from build123d import *

# Parameters (mm, degrees)
SKETCH1_W               = 55.5
SKETCH1_H               = 56
BOSS_EXTRUDE1_DEPTH     = 3
BOSS_EXTRUDE2_DEPTH     = 28
BOSS_EXTRUDE3_DEPTH     = 35
CUT_EXTRUDE3_DEPTH      = 61.495475037
CUT_EXTRUDE3_DEPTH_BACK = 61.495475037
SKETCH6_W               = 15.5
SKETCH6_H               = 56
BOSS_EXTRUDE4_DEPTH     = 0.6
SKETCH7_R               = 7.1
BOSS_EXTRUDE5_DEPTH     = 1.7
FILLET2_R               = 1


with BuildPart() as part:
    # Sketch1 → Boss-Extrude1 (new body)
    with BuildSketch(Plane(origin=(0, 0, 0), x_dir=(1, 0, 0), z_dir=(0, 1, 0))):
        Rectangle(SKETCH1_W, SKETCH1_H)
    extrude(amount=BOSS_EXTRUDE1_DEPTH)

    # Sketch3 → Boss-Extrude2 (add, symmetric)
    with BuildSketch(Plane.XY):
        Polygon((-27.75, 3), (-27.75, 40.8), (27.75, 40.8), (27.75, 3), (24.75, 3), (24.75, 37.8), (-24.75, 37.8), (-24.75, 3), align=None)
    extrude(amount=BOSS_EXTRUDE2_DEPTH, both=True)

    # Sketch4 → Boss-Extrude3 (add, symmetric)
    with BuildSketch(Plane.XY):
        Polygon((27.75, 40.8), (-27.75, 40.8), (-27.75, 37.5), (-27.75, 3), (-24.75, 3), (-24.75, 37.8), (24.75, 37.8), (24.75, 3), (27.75, 3), (27.75, 37.5), align=None)
    extrude(amount=BOSS_EXTRUDE3_DEPTH, both=True)

    # Sketch5 → Cut-Extrude3 (cut, two sides: drawn at the far end of the back side and taken through both)
    with BuildSketch(Plane(origin=(0, 0, 0), x_dir=(0, 0, -1), z_dir=(1, 0, 0)).offset(-CUT_EXTRUDE3_DEPTH_BACK)):
        with BuildLine():
            Line((-10.364011889, 35.8), (10.364011889, 35.8))
            ThreePointArc((10.364011889, 35.8), (6.080263232, 20.66392266), (7.526937591, 5))
            Line((7.526937591, 5), (-7.526937591, 5))
            ThreePointArc((-7.526937591, 5), (-6.080263232, 20.66392266), (-10.364011889, 35.8))
        make_face()
        with BuildLine():
            Line((-35, 37.5), (-35, 3))
            Line((-35, 3), (-28, 3))
            ThreePointArc((-28, 3), (-24.398228699, 21.690939105), (-35, 37.5))
        make_face()
        with BuildLine():
            Line((28, 3), (35, 3))
            Line((35, 3), (35, 37.5))
            ThreePointArc((35, 37.5), (24.398228699, 21.690939105), (28, 3))
        make_face()
    extrude(amount=CUT_EXTRUDE3_DEPTH + CUT_EXTRUDE3_DEPTH_BACK, mode=Mode.SUBTRACT)

    # Sketch6 → Boss-Extrude4 (add)
    with BuildSketch(Plane.XZ):
        Rectangle(SKETCH6_W, SKETCH6_H)
    extrude(amount=BOSS_EXTRUDE4_DEPTH)

    # Sketch7 → Boss-Extrude5 (add)
    with BuildSketch(Plane.XZ.offset(0.6)):
        with Locations(Location((0, 0, 0), (0, 0, 270))):
            Circle(SKETCH7_R)
    extrude(amount=BOSS_EXTRUDE5_DEPTH)

    # Fillet2
    fillet2_edges = [part.edges().sort_by_distance(p)[0] for p in [
        (27.75, 40.8, 0),
        (-27.75, 40.8, 0),
    ]]
    fillet(fillet2_edges, radius=FILLET2_R)


solid = part.part
Design review of the part built by this model. Coordinates are the model's own, in mm. A direction names the side the tool comes from. Coordinates: 2 decimals unless noted, no trailing zeros. Order: outer loops, then holes, each group sorted by start corner. A loop starts at its lowest first (then second) coordinate and runs counter-clockwise, first axis right, second up. Notation, with made-up numbers: (-32, 34.5) -> (-7, 34.5) arc R16 cw to (-7, 55.5) -> close; hole circle Ø11 at (74, 51.5). An arc over 180 degrees is marked (long way). Use one line per item in the form item = value. Start each with the question number.
(1) For faces 1 (the cylindrical face through (5.987, -1.438, -3.817)), 2 (the flat face through (0, 1, -28)), 3 (the flat face through (26, 35.8, 0)), 4 (the cylindrical face through (-26.271, 21.959, -24.454)), 5 (the flat face through (24.75, 21, 8)), list the 3-axis set-ups (+Z, -Z, +X, -X, +Y, -Y) from which the entire face can be reached by the end or side of a thin tool; tool diameter is ignored.
(2) Add section C-C on y = 19. State the section outline as (x, z) points, plus the area to 3 significant figures.
(3) Add section A-A on x = -14.5. State the section outline as (y, z) points.
(4) For probe 1 along Y at (x, z) = (10, -27); probe 2 along Y at (x, z) = (0, -16.5); probe 3 along X at (y, z) = (24, 21), list the stretches that pass through material, from the lowest coordinate up.
(5) Add section B-B on z = 0. State the section outline as (x, y) points.
(6) Insertion check: pin 1 (6 mm diameter, centred on y = 16.5, z = 3.5, fed in from +X); pin 2 (0.7 mm diameter, centred on y = -0.5, z = -3.5, fed in from -X); pin 3 (1.1 mm diameter, centred on x = 10, y = 1, fed in from -Z); pin 4 (1.5 mm diameter, centred on x = -25.5, z = -3.5, fed in from -Y). Each pin has a flat end and moves straight along its axis. Give the tip position at first contact, or say it passes through.
(7) The part is to be moulded in two halves that separate along Y. For faces 6 (the flat face through (0, 40.8, 0)), 7 (the flat face through (-26, 35.8, 0)), 8 (the cylindrical face through (26.229, 21.423, 24.345)), 9 (the flat face through (-18, 0, 0)), say which applies: +Y half, -Y half, draft (parallel to the pull), parting line (faces both ways), or undercut.
(8) Add section D-D on z = -15. State the section outline as (x, y) points.
Answer block:
q1.face_1 = -Y
q1.face_2 = -Z, +X, -X, -Y
q1.face_3 = +X, -X
q1.face_4 = -Z, +X, -X
q1.face_5 = +Z, -Z
q2.outline = (-27.75, -24) -> (-24.75, -24) -> (-24.75, -5.96) -> (-27.75, -5.96) -> close; (-27.75, 5.96) -> (-24.75, 5.96) -> (-24.75, 24) -> (-27.75, 24) -> close; (24.75, -24) -> (27.75, -24) -> (27.75, -5.96) -> (24.75, -5.96) -> close; (24.75, 5.96) -> (27.75, 5.96) -> (27.75, 24) -> (24.75, 24) -> close
q2.area = 217 mm²
q3.outline = (0, -28) -> (3, -28) -> (3, 28) -> (0, 28) -> close; (37.8, -35) -> (40.8, -35) -> (40.8, 35) -> (37.8, 35) -> close
q4.probe_1 = 0 to 3, 37.8 to 40.8
q4.probe_2 = -0.6 to 3, 37.8 to 40.8
q4.probe_3 = -27.75 to -24.75, 24.75 to 27.75
q5.outline = (-27.75, 0) -> (-7.75, 0) -> (-7.75, -0.6) -> (-7.1, -0.6) -> (-7.1, -2.3) -> (7.1, -2.3) -> (7.1, -0.6) -> (7.75, -0.6) -> (7.75, 0) -> (27.75, 0) -> (27.75, 5) -> (24.75, 5) -> (24.75, 3) -> (-24.75, 3) -> (-24.75, 5) -> (-27.75, 5) -> close; (-27.75, 35.8) -> (-24.75, 35.8) -> (-24.75, 37.8) -> (24.75, 37.8) -> (24.75, 35.8) -> (27.75, 35.8) -> (27.75, 39.8) arc R1 ccw to (26.75, 40.8) -> (-26.75, 40.8) arc R1 ccw to (-27.75, 39.8) -> close
q6.pin_1 = 27.75
q6.pin_2 = -7.75
q6.pin_3 = -28
q6.pin_4 = 0
q7.face_6 = +Y half
q7.face_7 = undercut
q7.face_8 = undercut
q7.face_9 = -Y half
q8.outline = (-27.75, 0) -> (-7.75, 0) -> (-7.75, -0.6) -> (7.75, -0.6) -> (7.75, 0) -> (27.75, 0) -> (27.75, 39.8) arc R1 ccw to (26.75, 40.8) -> (-26.75, 40.8) arc R1 ccw to (-27.75, 39.8) -> close; hole (-24.75, 3) -> (24.75, 3) -> (24.75, 37.8) -> (-24.75, 37.8) -> close
